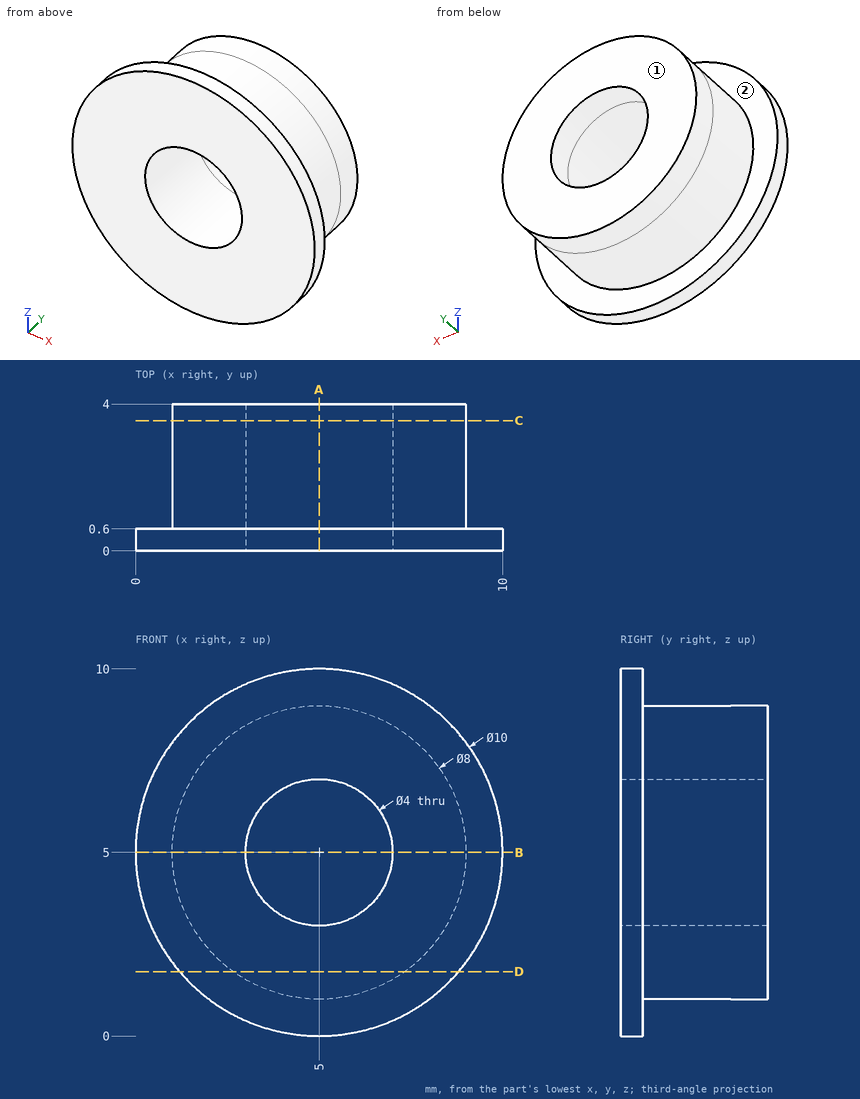
Input: dimensioned drawing with shaded views. Units: mm. Origin: part minimum x, y, z. A direction names the side the tool comes from. Coordinates: 2 decimals unless noted, no trailing zeros. Loops run counter-clockwise (first coordinate to the right, second up) from the corner with the lowest first, then second, coordinate; pieces in that order, holes last. Notation, with made-up numbers: M 27.5,-37 L 38.5,-37 A18 ccw 38.5,-19 Z; hole C 47,17 d6. An arc over 180 degrees is marked long. Use a Markdown table: item, result. Add a question column.
Q1. First-contact query: pin 1 (1.5 mm diameter, centred on x = 2.5, y = 1, fed in from -Z); pin 2 (1.5 mm diameter, centred on x = 3.5, y = 1, fed in from -Z). Flat tips, straight axial feed; report the tip coordinate or a pass-through.
Q2. Access query for the marked faces 1 and 2. Directions: +Z, -Z, +X, -X, +Y, -Y. A direction counts if a zero-diameter tool reaches every point of the face in a straight line with its end or side. Return the directions, or none.
Q3. Section query B-B, the plane z = 5. Return loops of the section in (x, y).
Q4. Section query A-A, the plane x = 5. Return loops of the section in (y, z), and give its area (3 significant figures).
Q5. Section query D-D, the plane z = 1.75. Return loops of the section in (x, y), and give its area (3 significant figures).
Q6. Section query C-C, the plane y = 3.55. Return loops of the section in (x, z), and give its area (3 significant figures).
Q7. Material intervals for L1, parallel to X at y = 1.25, z = 5; L2, parallel to X at y = 0.2, z = 3.25; L3, parallel to Y at x = 5, z = 9.5, sorted ascending.
Result:
| question | item | result |
|---|---|---|
| 1 | pin 1 | stops at z = 0.36 |
| 1 | pin 2 | stops at z = 0.08 |
| 2 | face 1 | +Z, -Z, +X, -X, +Y |
| 2 | face 2 | +Y |
| 3 | outline | M 0,0 L 3,0 L 3,4 L 1,4 L 1,0.6 L 0,0.6 Z; M 7,0 L 10,0 L 10,0.6 L 9,0.6 L 9,4 L 7,4 Z |
| 4 | outline | M 0,0 L 0.6,0 L 0.6,1 L 4,1 L 4,3 L 0,3 Z; M 0,7 L 4,7 L 4,9 L 0.6,9 L 0.6,10 L 0,10 Z |
| 4 | area | 17.2 mm2 |
| 5 | outline | M 1.2,0 L 8.8,0 L 8.8,0.6 L 7.33,0.6 L 7.33,4 L 2.67,4 L 2.67,0.6 L 1.2,0.6 Z |
| 5 | area | 20.4 mm2 |
| 6 | outline | C 5,5 d8; hole C 5,5 d4 |
| 6 | area | 37.7 mm2 |
| 7 | L1 | x = 1 to 3, 7 to 9 |
| 7 | L2 | x = 0.32 to 4.03, 5.97 to 9.68 |
| 7 | L3 | y = 0 to 0.6 |
